Check sheet for the modelled part. Datum: model origin and axes. Units: mm. A direction names the side the tool comes from. Give positions to 0.01 mm unless a question says otherwise; leave off trailing zeros. Order: outer loops, then holes, each group sorted by start corner. A loop starts at its lowest first (then second) coordinate and runs counter-clockwise, first axis right, second up.
Item 1: Access from +Z, -Z, +X, -X, +Y, -Y to the whole of each face (thin tool, end or side, straight path). Record for faces 5 (the flat face through (-33, 17, 150)), 6 (the flat face through (-33, 33, 0)), 7 (the flat face through (-48, 27.386, 302)).
Item 2: Release check for a two-part mould opening along Y. For faces 1 (the flat face through (-48, 32, 150)), 2 (the flat face through (-48, 37.386, 302)), 3 (the flat face through (-52.473, 39, 296)), 4 (the flat face through (-33, 22.386, 302)) record: released by +Y, released by -Y, zero draft, split by the parting line, or undercut.
Item 3: Material ranges on line 1 along X through (y, z) = (45, 450); line 2 along Y through (x, z) = (-44, 221); line 3 along Z through (x, y) = (-28, 15), recorded low to high.
Item 4: Sectioned sample at B-B on z = 420. Record the boundary of the cut face in (x, y), and give its area (3 significant figures).
Item 5: Sectioned sample at A-A on z = 111.5. Record the boundary of the cut face in (x, y).
Item 6: Gauge pin test, flat ends, axial feed: P1, Ø5.5, axis at x = -32.47, z = 450, coming from the +Y side; P2, Ø1, axis at x = -36, z = 402.5, coming from the -Y side. Record the tip position at first contact, or that the pin passes through.
from build123d import *

# Parameters (mm, degrees)
F0_W      = 40
F0_H      = 40
F1_DEPTH  = 600
F2_R      = 3
F3_DEPTH  = 12
F4_R      = 3
F5_DEPTH  = 12
F7_DEPTH  = 600
F8_R      = 3
F9_DEPTH  = 12
F10_DEPTH = 12
F11_R     = 3
F12_DEPTH = 12
F13_R     = 3
F14_DEPTH = 12
F16_W     = 10
F16_H     = 10
F17_DEPTH = 300
F18_DEPTH = 300


with BuildPart() as f1:
    # F0 (on Top) → F1 (new body)
    with BuildSketch(Plane.XY):
        with Locations((-32.4728810042, 32.3857110739)):
            Rectangle(F0_W, F0_H)
    extrude(amount=F1_DEPTH)

    # F2 (on face) → F3 (cut)
    with BuildSketch(Plane.YZ.offset(-12.4728810042)):
        with Locations((27.3857110739, 570)):
            Circle(F2_R)
    extrude(amount=-F3_DEPTH, mode=Mode.SUBTRACT)

    # F4 (on face) → F5 (cut)
    with BuildSketch(Plane(origin=(0, 52.3857110739, 0), x_dir=(-1, 0, 0), z_dir=(0, 1, 0))):
        with Locations((37.4728810042, 570)):
            Circle(F4_R)
    extrude(amount=-F5_DEPTH, mode=Mode.SUBTRACT)

    # F6 (on face) → F7 (cut)
    with BuildSketch(Plane.XY.offset(600)):
        with BuildLine():
            ThreePointArc((-47.5474812124, 12.3857110739), (-47.0872668168, 13.3390112528), (-46.9291592401, 14.3857110739))
            ThreePointArc((-46.9291592401, 14.3857110739), (-48.8190187951, 17.5198303656), (-52.4728810042, 17.3111108656))
            Line((-52.4728810042, 17.3111108656), (-52.4728810042, 12.3857110739))
            Line((-52.4728810042, 12.3857110739), (-47.5474812124, 12.3857110739))
        make_face()
    extrude(amount=-F7_DEPTH, mode=Mode.SUBTRACT)

    # F8 (on face) → F9 (cut)
    with BuildSketch(Plane.XY.offset(600)):
        with Locations((-32.4728810042, 32.3857110739)):
            Circle(F8_R)
    extrude(amount=-F9_DEPTH, mode=Mode.SUBTRACT)

    # F4 (on face) → F10 (cut)
    with BuildSketch(Plane(origin=(0, 52.3857110739, 0), x_dir=(-1, 0, 0), z_dir=(0, 1, 0))):
        with Locations((32.4728810042, 450)):
            Circle(F4_R)
    extrude(amount=-F10_DEPTH, mode=Mode.SUBTRACT)

    # F11 (on face) → F12 (cut)
    with BuildSketch(Plane(origin=(0, 52.3857110739, 0), x_dir=(-1, 0, 0), z_dir=(0, 1, 0))):
        with Locations((32.4728810042, 150)):
            Circle(F11_R)
    extrude(amount=-F12_DEPTH, mode=Mode.SUBTRACT)

    # F13 (on face) → F14 (cut)
    with BuildSketch(Plane.YZ.offset(-12.4728810042)):
        with Locations((32.3857110739, 100)):
            Circle(F13_R)
    extrude(amount=-F14_DEPTH, mode=Mode.SUBTRACT)

    # F16 (on offset) → F17 (cut)
    with BuildSketch(Plane.XY.offset(450)):
        with Locations((-47.4728810042, 32.3857110739)):
            Rectangle(F16_W, F16_H)
    extrude(amount=-F17_DEPTH, mode=Mode.SUBTRACT)

    # F16 (on offset) → F18 (cut)
    with BuildSketch(Plane.XY.offset(450)):
        with Locations((-32.4728810042, 17.3857110739)):
            Rectangle(F16_W, F16_H)
    extrude(amount=-F18_DEPTH, mode=Mode.SUBTRACT)


solid = f1.part
Report:
1. face 5: -Y
1. face 6: -Z, +X, -X, +Y, -Y
1. face 7: -X
2. face 1: undercut
2. face 2: undercut
2. face 3: zero draft
2. face 4: released by -Y
3. line 1: x = -52.47 to -35.47, -29.47 to -12.47
3. line 2: y = 12.39 to 27.39, 37.39 to 52.39
3. line 3: z = 0 to 150, 450 to 600
4. outline: (-52.47, 17.31) arc R3.54 cw to (-47.55, 12.39) - (-37.47, 12.39) - (-37.47, 22.39) - (-27.47, 22.39) - (-27.47, 12.39) - (-12.47, 12.39) - (-12.47, 52.39) - (-52.47, 52.39) - (-52.47, 37.39) - (-42.47, 37.39) - (-42.47, 27.39) - (-52.47, 27.39) - close
4. area: 1,370 mm2
5. outline: (-52.47, 17.31) arc R3.54 cw to (-47.55, 12.39) - (-12.47, 12.39) - (-12.47, 52.39) - (-52.47, 52.39) - close
6. P1: stops at y = 40.39
6. P2: stops at y = 22.39
